Autodesk Inventor part; units mm, degrees
ref_plane "YZ Plane" through (0, 0, 0) normal (1, 0, 0) x (0, 1, 0)
ref_plane "XZ Plane" through (0, 0, 0) normal (0, 1, 0) x (-1, 0, 0)
ref_plane "XY Plane" through (0, 0, 0) normal (0, 0, 1) x (1, 0, 0)
sketch "Sketch1" plane through (0, 0, 0) normal (0, 0, 1) x (1, 0, 0)
  circle A0 centre (0, 0) radius 19.05
  circle A1 centre (0, 0) radius 28.702
  dimension "d1" = 9.652
  dimension "d38" = 38.1
extrude "Extrusion1" add sketch "Sketch1" against normal blind 254 contours A0
extrude "Extrusion2" add sketch "Sketch1" along normal blind 6.35 contours A0 | A1
chamfer "Chamfer1" distance 3.175 angle 45 1 edges at (-19.05, 0, -254)
sketch "Sketch2" plane through (0, 0, 6.35) normal (0, 0, 1) x (1, 0, 0)
  circle A0 centre (0, 0) radius 28.702
  circle A1 centre (0, 0) radius 33.7566
  arc A2 (-68.8892, 89.446) -> (-67.2009, -88.2638) centre (-33.7441, 0.9169) ccw
  line L0 (-53.7761, -78.8636) -> (-67.2009, -88.2638)
  line L1 (0, -33.7566) -> (0, 33.7566)
  line L2 (-53.7761, 78.8636) -> (-53.7761, -78.8636)
  line L3 (-53.7761, 78.8636) -> (-68.8892, 89.446)
  line L4 (63.5, 33.7566) -> (-53.7761, 33.7566)
  line L5 (0, 0) -> (-53.7761, 0)
  line L6 (-146.05, 0) -> (-154.4505, 0)
  line L7 (63.5, -33.7566) -> (-53.7761, -33.7566)
  line L8 (0, 0) -> (63.5, 0)
  line L9 (63.5, 0) -> (63.5, -33.7566)
  line L10 (63.5, 0) -> (63.5, 33.7566)
  line L11 (-53.7761, 33.7566) -> (-123.154, 33.7566)
  line L12 (-53.7761, 0) -> (-128.9897, 0)
  line L13 (-53.7761, -33.7566) -> (-122.4589, -33.7566)
  dimension "d8" = 125
  dimension "d10" = 190.5
  dimension "d17" = 63.5
extrude "Extrusion10" add sketch "Sketch2" along normal blind 25.4 contours L8 L1 A0 | L8 A1 L1 A0 | A0 L1 L8 | A0 L1 A1 L8 | L1 L5 A0 | A0 L5 A1 L1 | L1 A1 L5 A0 | A0 L5 L1 | L8 L9 L7 A1 | A1 L4 L10 L8 | A1 L5 L2 L4 | L7 L2 L5 A1 | L2 L12 A2 L11 | L13 A2 L12 L2 | L2 L0 A2 L13
fillet "Fillet1" radius 25.4 4 edges at (-53.7761, -33.7566, 19.05) (63.5, -33.7566, 19.05) (63.5, 33.7566, 19.05) (-123.154, 33.7566, 19.05)
sketch "Sketch3" plane through (0, 0, 31.75) normal (0, 0, 1) x (1, 0, 0)
  circle A0 centre (0, 0) radius 28.702
  circle A1 centre (0, 0) radius 8.5985
  arc A2 (-103.1968, 33.7566) -> (-128.4523, 11.0619) centre (-103.1968, 8.3566) ccw
  arc A3 (-128.4523, 11.0619) -> (-67.2009, -88.2638) centre (-33.7441, 0.9169) ccw
  line L0 (-53.7761, -78.8636) -> (-67.2009, -88.2638)
  line L1 (-53.7761, -59.1566) -> (-53.7761, -78.8636)
  arc A4 (-28.3761, -33.7566) -> (-53.7761, -59.1566) centre (-28.3761, -59.1566) ccw
  line L2 (38.1, -33.7566) -> (-28.3761, -33.7566)
  arc A5 (38.1, -33.7566) -> (63.5, -8.3566) centre (38.1, -8.3566) ccw
  line L3 (63.5, 8.3566) -> (63.5, -8.3566)
  arc A6 (63.5, 8.3566) -> (38.1, 33.7566) centre (38.1, 8.3566) ccw
  line L4 (-103.1968, 33.7566) -> (38.1, 33.7566)
extrude "Extrusion5" add sketch "Sketch3" along normal blind 3.175 contours A0 | A1
extrude "Extrusion6" add sketch "Sketch3" along normal blind 6.35 contours A1
fillet "Fillet2" radius 25.4 1 edges at (-28.702, 0, 34.925)
sketch "Sketch4" plane through (0, 0, 31.75) normal (0, 0, 1) x (1, 0, 0)
  line L0 (63.5, 8.3566) -> (63.5, -8.3566)
  circle A0 centre (44.45, 0) radius 15.875
  circle A1 centre (44.45, 0) radius 9.525
  arc A2 (-28.702, 0) -> (28.702, 0) centre (0, 0) ccw
  arc A3 (28.702, 0) -> (-28.702, 0) centre (0, 0) ccw
  arc A4 (-103.1968, 33.7566) -> (-128.4523, 11.0619) centre (-103.1968, 8.3566) ccw
  arc A5 (-128.4523, 11.0619) -> (-67.2009, -88.2638) centre (-33.7441, 0.9169) ccw
  line L1 (-53.7761, -78.8636) -> (-67.2009, -88.2638)
  line L2 (-53.7761, -59.1566) -> (-53.7761, -78.8636)
  arc A6 (-28.3761, -33.7566) -> (-53.7761, -59.1566) centre (-28.3761, -59.1566) ccw
  line L3 (38.1, -33.7566) -> (-28.3761, -33.7566)
  arc A7 (38.1, -33.7566) -> (63.5, -8.3566) centre (38.1, -8.3566) ccw
  line L4 (63.5, 8.3566) -> (63.5, -8.3566)
  arc A8 (63.5, 8.3566) -> (38.1, 33.7566) centre (38.1, 8.3566) ccw
  line L5 (-103.1968, 33.7566) -> (38.1, 33.7566)
  dimension "d24" = 19.05
  dimension "d25" = 31.75
  dimension "d26" = 19.05
extrude "Extrusion7" add sketch "Sketch4" along normal blind 120.65 contours A1
extrude "Extrusion8" add sketch "Sketch4" along normal blind 114.3 contours A0 A2 A3 | A3 A2 A0 picked at (58.0643, -1.2262) picked at (28.6234, 0)
fillet "Fillet3" radius 3.175 2 edges at (45.2559, 15.8545, 31.75) (45.2559, -15.8545, 31.75)
sketch "Sketch5" plane through (0, 0, -254) normal (0, 0, -1) x (-1, 0, 0)
  circle A0 centre (0, 0) radius 15.875
  line L0 (6.35, 5.9176) -> (31.75, 5.9176)
  line L1 (31.75, 5.9176) -> (31.75, -6.7824)
  line L2 (31.75, -6.7824) -> (6.35, -6.7824)
  line L3 (6.35, -6.7824) -> (6.35, 5.9176)
  dimension "d32" = 12.7
  dimension "d33" = 25.4
  dimension "d34" = 6.35
extrude "Extrusion9" cut sketch "Sketch5" against normal blind 76.2 contours A0 L2 L3 L0 | A0 L0 L1 L2 picked at (9.525, -0.2883)
fillet "Fillet4" radius 3.175 2 edges at (-12.0759, -6.7824, -177.8) (-12.2288, 5.9176, -177.8)
equation "\"d9\" = d8"
equation "\"d12\" = d11"
properties part number "Crankshaft" material "Steel, High Strength Low Alloy"
Design review of the part built by this model. Coordinates are the model's own, in mm. A direction names the side the tool comes from. Give positions to 0.01 mm unless a question says otherwise; leave off trailing zeros. Write each loop counter-clockwise with the first axis right and the second up, starting at its lowest first coordinate (ties: lowest second). Pieces come first, ordered by that corner, then holes. Notation, with made-up numbers: (28.5, 81) -> (71.5, 81) arc R10 ccw to (71.5, 95) -> close; hole circle Ø5 at (67, 69.25). An arc over 180 degrees is marked (long way). Answer in a Markdown table with one row per item.
(1) Consider section C-C (y = -50). State the section outline as (x, z) points, then the cut area to 3 significant figures.
Results:
| item | result |
|---|---|
| outline | (-114.24, 6.35) -> (-52.07, 6.35) -> (-52.07, 31.75) -> (-114.24, 31.75) -> close |
| area | 1,580 mm2 |
(2) Consider section D-D (z = -52.5). State the section outline as (x, y) points.
Results:
| item | result |
|---|---|
| outline | circle Ø38.1 at (0, 0) |
(3) For faces 4 (the cylindrical face through (-119.98, 27.42, 19.23)), 5 (the flat face through (6, -19, 0)), 6 (the flat face through (-12, -6.782, -218)), 7 (the flat face through (44, -10, 146.05)), 8 (the flat face through (-53.776, -69, 19)), list the 3-axis set-ups (+Z, -Z, +X, -X, +Y, -Y) from which the entire face can be reached by the end or side of a thin tool; tool diameter is ignored.
Results:
| item | result |
|---|---|
| face 4 | +Z, -Z, -X, +Y |
| face 5 | -Z |
| face 6 | -Z, -X |
| face 7 | +Z |
| face 8 | +Z, -Z, +X, -Y |
(4) Mouldability with a two-part tool opening along X and no side actions: class faces 1 (the flat face through (7, -7, 34.925)), 2 (the flat face through (-6.35, -1, -216)), 3 (the cylindrical face through (-6.22, 28.02, 3.13)) as +X half, -X half, draft (parallel to the pull), parting line (faces both ways), or undercut.
Results:
| item | result |
|---|---|
| face 1 | undercut |
| face 2 | -X half |
| face 3 | parting line |
(5) Consider section A-A (x = 44.45). State the section outline as (y, z) points (3 decimals).
Results:
| item | result |
|---|---|
| outline | (-32.95, 6.35) -> (32.95, 6.35) -> (32.95, 31.75) -> (19.05, 31.75) arc R3.175 cw to (15.875, 34.925) -> (15.875, 146.05) -> (9.525, 146.05) -> (9.525, 152.4) -> (-9.525, 152.4) -> (-9.525, 146.05) -> (-15.875, 146.05) -> (-15.875, 34.925) arc R3.175 cw to (-19.05, 31.75) -> (-32.95, 31.75) -> close |
(6) To check wall thickness, follow probe 1 along Z at (x, y) = (-44, -2); probe 2 along Y at (x, z) = (43.5, 50); probe 3 along Y at (x, z) = (12.5, 26). State the ranges of each line that lie inside material, in increasing order.
Results:
| item | result |
|---|---|
| probe 1 | 6.35 to 31.75 |
| probe 2 | -15.85 to 15.85 |
| probe 3 | -33.76 to 33.76 |
(7) Consider section B-B (z = 78.5). State the section outline as (x, y) points (3 decimals).
Results:
| item | result |
|---|---|
| outline | circle Ø31.75 at (44.45, 0) |
(8) Clearance check with flat-ended pins moving along their axes: pin 1 (10 mm diameter, centred on y = 2.5, z = -215.5, fed in from -X); pin 2 (3 mm diameter, centred on y = -3, z = -118, fed in from -X); pin 3 (3 mm diameter, centred on x = -43.5, y = 4.5, fed in from -Z). State where each tip first meets the part, or that it passes through.
Results:
| item | result |
|---|---|
| pin 1 | x = -18.11 |
| pin 2 | x = -18.99 |
| pin 3 | z = 6.35 |
